Build history of the part. All positions in model axes, mm. A direction names the side the tool comes from. Give positions to 0.01 mm unless a question says otherwise; leave off trailing zeros. Loops run counter-clockwise (first coordinate to the right, second up) from the corner with the lowest first, then second, coordinate; pieces in that order, holes last. Notation, with made-up numbers: (38.5, 28) -> (51.5, 28) arc R11 ccw to (51.5, 43) -> close; hole circle Ø8 at (80.5, 30.25). An arc over 180 degrees is marked (long way). Answer as a JSON object with one key per item and string values. Group by question number.
Q1. Tool access for faces 5 (the flat face through (25.044, 16.656, 13.86)), 6 (the flat face through (0, 0, 4)), 7 (the flat face through (-25.756, -19.774, 13.86)), 8 (the flat face through (33, -6.25, 1)), 9 (the flat face through (-25.044, -16.656, 13.86)): list every direction of +Z, -Z, +X, -X, +Y, -Y with a clear straight run to the whole face (end or side of a thin tool).
Q2. Drop flat-ended pins along their axis: pin 1 (10.5 mm diameter, centred on x = -19.5, y = -36.5, fed in from +Z); pin 2 (1 mm diameter, centred on x = -35, z = 12, fed in from -Y); pin 3 (1 mm diameter, centred on x = 28, z = 17, fed in from +Y). Give the stop position or say it passes through.
Q3. Band-saw the part on B-B, the plane z = 15.25. Write the cut outline in (x, y).
Q4. Wall check: probe 1 along Z at (x, y) = (-38, 23); probe 2 along Y at (x, z) = (9, 5.5); probe 3 along Y at (x, z) = (-11, 7.25). Give the ranges that are in metal, low to high. Write a range as from..to.
Q5. Two-plate mould, pull along X, no slides. Class faces 1 (the flat face through (25.756, 19.774, 13.86)), 2 (the flat face through (25.04, -19.68, 13.86)), 3 (the flat face through (27, 8, 2.5)), 4 (the cylindrical face through (-4.628, -0.247, 3.26)): pulls with the +X half, pulls with the -X half, needs draft (parallel to the pull), parting line crosses it, or undercut.
Q6. Band-saw the part on C-C, the plane x = -18. Write the cut outline in (y, z), plus the area to 3 significant figures.
Q7. Band-saw the part on D-D, the plane x = -6.5. Write the cut outline in (y, z).
Q8. Band-saw the part on A-A, the plane y = 0. Write the cut outline in (x, z) (3 decimals), plus the area to 3 significant figures.
from build123d import *

# Parameters (mm, degrees)
F0_W     = 101.6
F0_H     = 101.6
F1_DEPTH = 4
F3_DEPTH = 1.5
F5_DEPTH = 25.4
F7_DEPTH = 20


with BuildPart() as f1:
    # F0 (on Top) → F1 (new body)
    with BuildSketch(Plane.XY):
        Rectangle(F0_W, F0_H)
    extrude(amount=F1_DEPTH)

    # F2 (on face) → F3 (cut)
    with BuildSketch(Plane.XY.offset(4)):
        with BuildLine():
            Line((15.875, -11.25), (50.8, -11.25))
            Line((50.8, -11.25), (50.8, 11.25))
            Line((50.8, 11.25), (15.875, 11.25))
            ThreePointArc((15.875, 11.25), (4.625, 0), (15.875, -11.25))
        make_face()
        with BuildLine():
            Line((-50.8, -11.25), (-15.875, -11.25))
            ThreePointArc((-15.875, -11.25), (-4.625, 0), (-15.875, 11.25))
            Line((-15.875, 11.25), (-50.8, 11.25))
            Line((-50.8, 11.25), (-50.8, -11.25))
        make_face()
    extrude(amount=-F3_DEPTH, mode=Mode.SUBTRACT)

    # F4 (on face) → F5 (cut)
    with BuildSketch(Plane.XY.offset(2.5)):
        with BuildLine():
            ThreePointArc((-15.875, -6.25), (-9.625, 0), (-15.875, 6.25))
            Line((-15.875, 6.25), (-50.8, 6.25))
            Line((-50.8, 6.25), (-50.8, -6.25))
            Line((-50.8, -6.25), (-15.875, -6.25))
        make_face()
        with BuildLine():
            ThreePointArc((15.875, 6.25), (9.625, 0), (15.875, -6.25))
            Line((15.875, -6.25), (50.8, -6.25))
            Line((50.8, -6.25), (50.8, 6.25))
            Line((50.8, 6.25), (15.875, 6.25))
        make_face()
    extrude(amount=-F5_DEPTH, mode=Mode.SUBTRACT)

    # F6 (on face) → F7 (join)
    with BuildSketch(Plane.XY.offset(4)):
        Polygon((0, -13.405257), (-50.8, -20), (-50.8, -23.025173), (0, -16.430431), (50.8, -23.025173), (50.8, -20), align=None)
        Polygon((-50.8, 23.025173), (-50.8, 20), (0, 13.405257), (50.8, 20), (50.8, 23.025173), (0, 16.430431), align=None)
    extrude(amount=F7_DEPTH)


solid = f1.part
Worked answers:
{
 "1": {"face 5": "+Z, +X", "face 6": "+Z", "face 7": "+Z, -Y", "face 8": "+Z, -Z, +X", "face 9": "+Z, -X"},
 "2": {"pin 1": "z = 4", "pin 2": "y = -21.04", "pin 3": "y = 20.13"},
 "3": {"outline": "(-50.8, -23.03) -> (0, -16.43) -> (50.8, -23.03) -> (50.8, -20) -> (0, -13.41) -> (-50.8, -20) -> close; (-50.8, 20) -> (0, 13.41) -> (50.8, 20) -> (50.8, 23.03) -> (0, 16.43) -> (-50.8, 23.03) -> close"},
 "4": {"probe 1": "0..4", "probe 2": "-17.6..-14.57, 14.57..17.6", "probe 3": "-17.86..-14.83, 14.83..17.86"},
 "5": {"face 1": "undercut", "face 2": "undercut", "face 3": "needs draft", "face 4": "pulls with the -X half"},
 "6": {"outline": "(-50.8, 0) -> (-6.25, 0) -> (-6.25, 2.5) -> (-11.25, 2.5) -> (-11.25, 4) -> (-15.74, 4) -> (-15.74, 24) -> (-18.77, 24) -> (-18.77, 4) -> (-50.8, 4) -> close; (6.25, 0) -> (50.8, 0) -> (50.8, 4) -> (18.77, 4) -> (18.77, 24) -> (15.74, 24) -> (15.74, 4) -> (11.25, 4) -> (11.25, 2.5) -> (6.25, 2.5) -> close", "area": "462 mm2"},
 "7": {"outline": "(-50.8, 0) -> (50.8, 0) -> (50.8, 4) -> (17.27, 4) -> (17.27, 24) -> (14.25, 24) -> (14.25, 4) -> (6.22, 4) -> (6.22, 2.5) -> (-6.22, 2.5) -> (-6.22, 4) -> (-14.25, 4) -> (-14.25, 24) -> (-17.27, 24) -> (-17.27, 4) -> (-50.8, 4) -> close"},
 "8": {"outline": "(-9.625, 0) -> (9.625, 0) -> (9.625, 2.5) -> (4.625, 2.5) -> (4.625, 4) -> (-4.625, 4) -> (-4.625, 2.5) -> (-9.625, 2.5) -> close", "area": "62.0 mm2"}
}
